Check sheet for the drawn part. Datum: minimum x, y, z corner. Units: mm. A direction names the side the tool comes from. Round coordinates to 2 decimals unless told otherwise and drop trailing zeros. Write each loop counter-clockwise with the first axis right and the second up, starting at its lowest first coordinate (ties: lowest second). Pieces come first, ordered by that corner, then holes. Notation, with made-up numbers: M 13.25,77 L 70.25,77 A17 cw 70.25,109 Z; hole C 80,68 d6. An arc over 180 degrees is marked long. One line per item, written item: value.
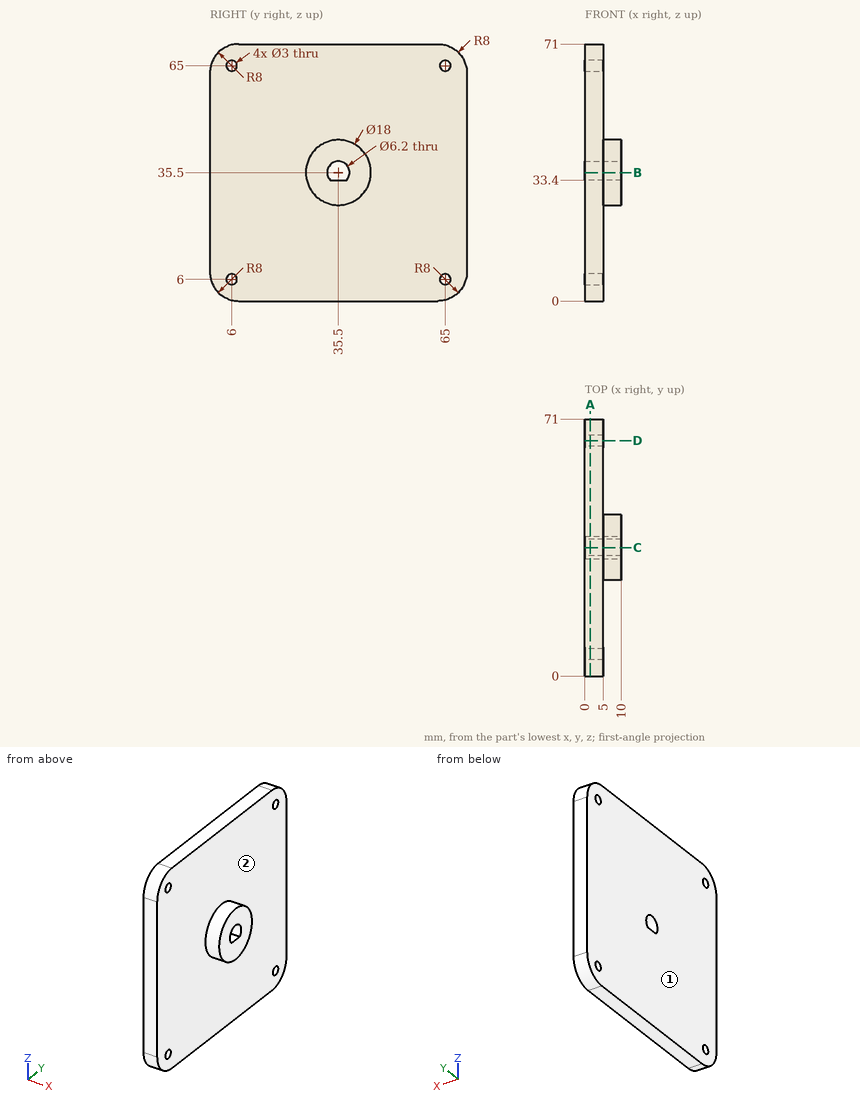
Q1. Depth check by flat-ended pin: P1, Ø12, axis at y = 30.5, z = 7, coming from the +X side; P2, Ø2.5, axis at y = 65, z = 65, coming from the +X side; P3, Ø5, axis at y = 35.5, z = 35.5, coming from the -X side. Enter the tip coordinate at first touch or a pass-through.
Completed:
P1: x = 5
P2: through
P3: x = 0
Q2. Access from +Z, -Z, +X, -X, +Y, -Y to the whole of each face (thin tool, end or side, straight path). Record for the marked faces 1 and 2.
Completed:
face 1: +Z, -Z, -X, +Y, -Y
face 2: +X
Q3. Sectioned sample at D-D on y = 65. Enter the section's corners in (x, z).
Completed:
outline: M 0,0.25 L 5,0.25 L 5,4.5 L 0,4.5 Z; M 0,7.5 L 5,7.5 L 5,63.5 L 0,63.5 Z; M 0,66.5 L 5,66.5 L 5,70.75 L 0,70.75 Z
Q4. Sectioned sample at A-A on x = 1.5. Enter the section's corners in (y, z).
Completed:
outline: M 0,8 A8 ccw 8,0 L 63,0 A8 ccw 71,8 L 71,63 A8 ccw 63,71 L 8,71 A8 ccw 0,63 Z; hole C 6,6 d3; hole C 6,65 d3; hole M 33.22,33.4 L 37.78,33.4 A3.1 ccw long Z; hole C 65,6 d3; hole C 65,65 d3
Q5. Sectioned sample at B-B on z = 35.5. Enter the section's corners in (x, y).
Completed:
outline: M 0,0 L 5,0 L 5,26.5 L 10,26.5 L 10,32.4 L 0,32.4 Z; M 0,38.6 L 10,38.6 L 10,44.5 L 5,44.5 L 5,71 L 0,71 Z
Q6. Sectioned sample at C-C on y = 35.5. Enter the section's corners in (x, z).
Completed:
outline: M 0,0 L 5,0 L 5,26.5 L 10,26.5 L 10,33.4 L 0,33.4 Z; M 0,38.6 L 10,38.6 L 10,44.5 L 5,44.5 L 5,71 L 0,71 Z
Q7. Scan lines: line 1 (Y direction, x = 2.5, z = 65); line 2 (Y direction, x = 2.75, z = 35.5); line 3 (X direction, y = 27, z = 25). Record each from-to range of solid material in increasing order. Write a range as [from, to].
Completed:
line 1: [0.25, 4.5], [7.5, 63.5], [66.5, 70.75]
line 2: [0, 32.4], [38.6, 71]
line 3: [0, 5]
